Can you work these out from the model? Positions are in its coordinate system, mm. A direction names the side the tool comes from. Round coordinates to 2 decimals unless told otherwise and drop trailing zeros. Order: outer loops, then holes, each group sorted by start corner. A loop starts at its lowest first (then second) coordinate and runs counter-clockwise, first axis right, second up. Notation, with made-up numbers: M 30.5,70.5 L 83.5,70.5 A12 ccw 83.5,81.5 Z; hole C 37.25,81.5 d10. An arc over 180 degrees is marked long. Answer as a JSON object with one key per item and string values. Group by question number.
from build123d import *

# Parameters (mm, degrees)
F0_R     = 9.525
F1_DEPTH = 127
F2_W     = 133.35
F2_H     = 3.175
F2_W_2   = 28.575
F3_DEPTH = 12.7
F4_SIZE  = 1.524
F5_R     = 3.17499


# Not quite as in the source:
# - a fillet or chamfer is up to 0.001 mm smaller than in the source, because OpenCascade refuses the exact size


with BuildPart() as f1:
    # F0 (on Front) → F1 (new body, symmetric)
    with BuildSketch(Plane.XZ):
        Circle(F0_R)
    extrude(amount=F1_DEPTH, both=True)

    # F2 (on Right) → F3 (cut, symmetric)
    with BuildSketch(Plane.YZ):
        with Locations((0, 7.9375)):
            Rectangle(F2_W, F2_H)
        with Locations((-112.7125, 7.9375)):
            Rectangle(F2_W_2, F2_H)
        with Locations((112.7125, 7.9375)):
            Rectangle(F2_W_2, F2_H)
    extrude(amount=F3_DEPTH, both=True, mode=Mode.SUBTRACT)

    # F4
    f4_edges = [f1.edges().sort_by_distance(p)[0] for p in [
        (-3.39873, -127, -8.897992),
        (-3.39873, 127, -8.897992),
    ]]
    chamfer(f4_edges, length=F4_SIZE)

    # F5 (radius 3.175 in the source; OpenCascade refuses exactly that, so slightly less here)
    f5_edges = [f1.edges().sort_by_distance(p)[0] for p in [
        (0, -98.425, 6.35),
        (0, 66.675, 6.35),
        (0, 98.425, 6.35),
        (0, -66.675, 6.35),
    ]]
    fillet(f5_edges, radius=F5_R)


solid = f1.part
Item 1: If we mould it in two halves opening along Y, with no side actions, what happens to faces 3 (the face through (0, -1, 6.35)), 4 (the face through (-0.287, 126.757, -8.239)), 5 (the face through (0, 114, 6.35)), 6 (the face through (-0.287, -126.757, -8.239))? For each: +Y half, -Y half, draft (parallel to the pull), parting line (faces both ways), or undercut.
Item 2: On a 3-axis mill with a long thin cutter (end or side, diameter ignored), from which of +Z, -Z, +X, -X, +Y, -Y can I reach the whole of each face in a straight line? I mean faces 1 (the face through (-2.06, -1.76, -9.3)), 2 (the face through (0, -114, 6.35)). Say none if no direction works.
Item 3: I'm going to push flat-ended pins straight in: pin 1 Ø3 at (y, z) = (-8.5, 5.5) entering from -X; pin 2 Ø5 at (y, z) = (-42.5, -6) entering from -X; pin 3 Ø3 at (y, z) = (44.5, -6) entering from +X (3 decimals). Where does each tip first touch, or does it pass through?
Item 4: I need wall thicknesses on line 1 (X direction, y = -58.5, z = 0.25); line 2 (Y direction, x = 1, z = 7); line 3 (Z direction, x = 0.5, y = 4.5). Which ranges of each line are inside material? Lowest first, please.
Item 5: Suppose I cut it at B-B, the plane y = 88.5. Write out the boundary of the cut face in (x, z) (3 decimals), and give its area (3 significant figures).
Item 6: Suppose I cut it at A-A, the plane y = -25.5. Write out the boundary of the cut face in (x, z) (3 decimals).
Computed:
{
 "1": {"face 3": "undercut", "face 4": "+Y half", "face 5": "draft", "face 6": "-Y half"},
 "2": {"face 1": "+Y, -Y", "face 2": "+Z, +X, -X, -Y"},
 "3": {"pin 1": "stops at x = -8.64", "pin 2": "stops at x = -8.86", "pin 3": "stops at x = 8.395"},
 "4": {"line 1": "x = -9.52 to 9.52", "line 2": "y = -99.68 to -65.42, 65.42 to 99.68", "line 3": "z = -9.51 to 6.35"},
 "5": {"outline": "C 0,0 d19.05", "area": "285 mm^2"},
 "6": {"outline": "M -7.1,6.35 A9.525 ccw long 7.1,6.35 Z"}
}
